from build123d import *

# Parameters (mm, degrees)
ESQUISSE1_R        = 1.5
ESQUISSE1_R_2      = 0.5
BOSS_EXTRU_1_DEPTH = 2
ESQUISSE2_R        = 4.1
ESQUISSE2_R_2      = 2.5
BOSS_EXTRU_2_DEPTH = 3


with BuildPart() as part:
    # Esquisse1 → Boss.-Extru.1 (new body)
    with BuildSketch(Plane.XY):
        with BuildLine():
            Line((-16.337044695, 1.536467752), (-4.650806382, 4.1))
            ThreePointArc((-4.650806382, 4.1), (0, 6.2), (4.650806382, 4.1))
            Line((4.650806382, 4.1), (16.337044695, 1.536467752))
            ThreePointArc((16.337044695, 1.536467752), (17.573001042, 0), (16.337044695, -1.536467752))
            Line((16.337044695, -1.536467752), (4.650806382, -4.1))
            ThreePointArc((4.650806382, -4.1), (0, -6.2), (-4.650806382, -4.1))
            Line((-4.650806382, -4.1), (-16.337044695, -1.536467752))
            ThreePointArc((-16.337044695, -1.536467752), (-17.573001042, 0), (-16.337044695, 1.536467752))
        make_face()
        Circle(ESQUISSE1_R, mode=Mode.SUBTRACT)
        with Locations((7, 0)):
            Circle(ESQUISSE1_R_2, mode=Mode.SUBTRACT)
        with Locations((16, 0)):
            Circle(ESQUISSE1_R_2, mode=Mode.SUBTRACT)
        with Locations((13, 0)):
            Circle(ESQUISSE1_R_2, mode=Mode.SUBTRACT)
        with Locations((10, 0)):
            Circle(ESQUISSE1_R_2, mode=Mode.SUBTRACT)
        with Locations((-16, 0)):
            Circle(ESQUISSE1_R_2, mode=Mode.SUBTRACT)
        with Locations((-13, 0)):
            Circle(ESQUISSE1_R_2, mode=Mode.SUBTRACT)
        with Locations((-10, 0)):
            Circle(ESQUISSE1_R_2, mode=Mode.SUBTRACT)
        with Locations((-7, 0)):
            Circle(ESQUISSE1_R_2, mode=Mode.SUBTRACT)
    extrude(amount=BOSS_EXTRU_1_DEPTH)

    # Esquisse2 → Boss.-Extru.2 (add)
    with BuildSketch(Plane.XY.offset(2)):
        Circle(ESQUISSE2_R)
        Circle(ESQUISSE2_R_2, mode=Mode.SUBTRACT)
    extrude(amount=BOSS_EXTRU_2_DEPTH)


solid = part.part
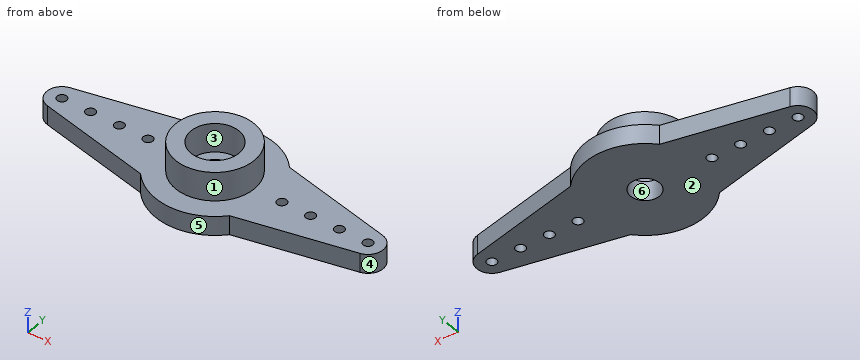
Verification items for the finished model (mm, model axes). Face numbers are marked on the shaded views. A direction names the side the tool comes from. Coordinates: 2 decimals unless noted, no trailing zeros. Loops run counter-clockwise (first coordinate to the right, second up) from the corner with the lowest first, then second, coordinate; pieces in that order, holes last. Notation, with made-up numbers: (49, 48.5) -> (61, 48.5) arc R13 cw to (61, 58.5) -> close; hole circle Ø5 at (30, 48.5). An arc over 180 degrees is marked (long way). Answer as CSV lines item,"result".
1) Cross-section at A-A, the plane x = 0. Record the cut outline in (y, z), then the cut area to 3 significant figures.
Found:
outline,"(-6.2, 0) -> (-1.5, 0) -> (-1.5, 2) -> (-2.5, 2) -> (-2.5, 5) -> (-4.1, 5) -> (-4.1, 2) -> (-6.2, 2) -> close; (1.5, 0) -> (6.2, 0) -> (6.2, 2) -> (4.1, 2) -> (4.1, 5) -> (2.5, 5) -> (2.5, 2) -> (1.5, 2) -> close"
area,"28.4 mm2"
2) Tool access check on the marked faces 1 and 2. Record the directions out of +Z, -Z, +X, -X, +Y, -Y that give a thin tool (end or side, any length) a straight path to the whole face; none if there is none.
Found:
face 1,"+Z"
face 2,"-Z, +X, -X, +Y, -Y"
3) Depth check by flat-ended pin: pin 1 (2 mm diameter, centred on x = 13.5, z = 1.5, fed in from +Y); pin 2 (4.5 mm diameter, centred on x = 0, y = 0, fed in from +Z); pin 3 (1 mm diameter, centred on y = -2.5, z = 4.5, fed in from -X). Enter the tip coordinate at first touch or a pass-through.
Found:
pin 1,"stops at y = 2.38"
pin 2,"stops at z = 2"
pin 3,"stops at x = -3.58"
4) Release check for a two-part mould opening along Y. For the marked faces 3, 4, 5 and 6 record: +Y half, -Y half, draft (parallel to the pull), parting line (faces both ways), or undercut.
Found:
face 3,"undercut"
face 4,"parting line"
face 5,"-Y half"
face 6,"undercut"
5) Thickness scan on L1, parallel to Y at x = 0, z = 1.55; L2, parallel to Z at x = -6, y = 1; L3, parallel to X at y = 2, z = 2.35. Record the ranges inside material, lowest first. Write a range as from..to.
Found:
L1,"y = -6.2..-1.5, 1.5..6.2"
L2,"z = 0..2"
L3,"x = -3.58..-1.5, 1.5..3.58"
6) Cross-section at D-D, the plane z = 3.9. Record the cut outline in (x, y).
Found:
outline,"circle Ø8.2 at (0, 0); hole circle Ø5 at (0, 0)"
7) Cross-section at B-B, the plane z = 0.7. Count the separate pieces of the cut face and the enclosed holes in it, then the cut area to 3 significant figures.
Found:
separate pieces,"1"
enclosed holes,"9"
area,"227 mm2"
